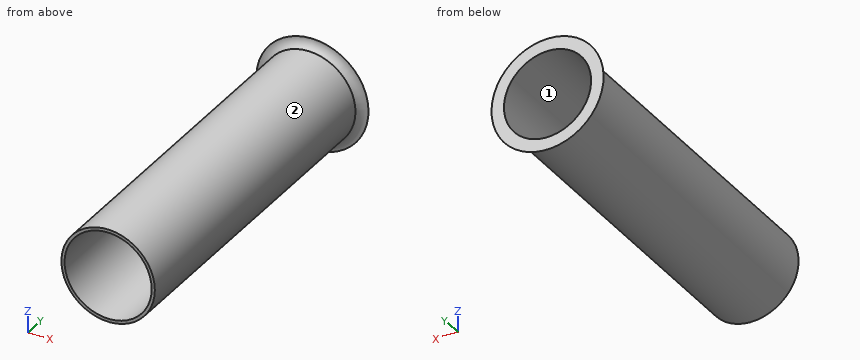
from build123d import *

# Parameters (mm, degrees)
F0_R     = 15
F1_DEPTH = 111
F2_R     = 14
F3_DEPTH = 111


with BuildPart() as f1:
    # F0 (on Front) → F1 (new body)
    with BuildSketch(Plane.XZ):
        Circle(F0_R)
    extrude(amount=F1_DEPTH)

    # F2 (on face) → F3 (cut)
    with BuildSketch(Plane.XZ.offset(111)):
        Circle(F2_R)
    extrude(amount=-F3_DEPTH, mode=Mode.SUBTRACT)

    # F4 (on Right) → F5 (revolve)
    with BuildSketch(Plane.YZ):
        with BuildLine():
            Line((-2, 15), (0, 15))
            Line((0, 15), (0, 18))
            ThreePointArc((0, 18), (-0.559736, 16.206491), (-2, 15))
        make_face()
    revolve(axis=Axis((0, -111, 0), (0, -1, 0)))


solid = f1.part
Geometry: final body of the model. Coordinates: model frame, mm. Face numbers are marked on the shaded views. Give positions to 0.01 mm unless a question says otherwise; leave off trailing zeros. Loops run counter-clockwise (first coordinate to the right, second up) from the corner with the lowest first, then second, coordinate; pieces in that order, holes last. Notation, with made-up numbers: M 80.5,-11 L 106.5,-11 A26 cw 106.5,25 Z; hole C -12,35 d9. An arc over 180 degrees is marked long. Put each result on its own line as item: value. Start each with the question number.
1) Cut plane C-C (y = -54). Output: boundary loops of the cut face in (x, z), then the cut area to 3 significant figures.
2) Ray query, line 1 along Z through (x, y) = (0, -22); line 2 along X through (y, z) = (-106, 9); line 3 along X through (y, z) = (-58.5, -4.5). Return the intervals inside material, ascending.
3) Pull-direction query (Z, two-part tool) for the marked faces 1 and 2; classes: pulls with the +Z half, pulls with the -Z half, needs draft (parallel to the pull), parting line crosses it, or undercut.
4) Contact query for flat-ended pins moving along their axis: pin 1 (8 mm diameter, centred on y = -30.5, z = 9.5, fed in from -X); pin 2 (2 mm diameter, centred on x = 11, y = -68.5, fed in from +Z); pin 3 (6 mm diameter, centred on y = -27.5, z = 12.5, fed in from -X); pin 4 (3 mm diameter, centred on x = 14.5, z = -4.5, fed in from -Y). Output: stop coordinate, or through.
5) Cut plane A-A (x = 0). Output: boundary loops of the cut face in (y, z), then the cut area to 3 significant figures.
6) Cut plane B-B (z = 0). Output: boundary loops of the cut face in (x, y).
Verdict:
1. outline: C 0,0 d30; hole C 0,0 d28
1. area: 91.1 mm2
2. line 1: -15 to -14, 14 to 15
2. line 2: -12 to -10.72, 10.72 to 12
2. line 3: -14.31 to -13.26, 13.26 to 14.31
3. face 1: undercut
3. face 2: parting line crosses it
4. pin 1: x = -13.96
4. pin 2: z = 11.18
4. pin 3: x = -11.61
4. pin 4: y = -111
5. outline: M -111,-15 L -2,-15 A3.34 cw 0,-18 L 0,-14 L -111,-14 Z; M -111,14 L 0,14 L 0,18 A3.34 cw -2,15 L -111,15 Z
5. area: 225 mm2
6. outline: M -18,0 A3.34 cw -15,-2 L -15,-111 L -14,-111 L -14,0 Z; M 14,-111 L 15,-111 L 15,-2 A3.34 cw 18,0 L 14,0 Z
